Geometry: final body of the model. Coordinates: model frame, mm. A direction names the side the tool comes from. Coordinates: 2 decimals unless noted, no trailing zeros. Write each loop counter-clockwise with the first axis right and the second up, starting at its lowest first coordinate (ties: lowest second). Pieces come first, ordered by that corner, then holes. Notation, with made-up numbers: (70, 45) - (103, 45) arc R13 cw to (103, 60) - close; hole circle Ø4 at (-15, 44.25). An arc over 180 degrees is marked (long way). Put each result on its own line as item: value.
Autodesk Inventor part; units mm, degrees
ref_plane "YZ Plane" through (0, 0, 0) normal (1, 0, 0) x (0, 1, 0)
ref_plane "XZ Plane" through (0, 0, 0) normal (0, 1, 0) x (-1, 0, 0)
ref_plane "XY Plane" through (0, 0, 0) normal (0, 0, 1) x (1, 0, 0)
sketch "Sketch1" plane through (0, 0, 0) normal (0, 1, 0) x (-1, 0, 0)
  line L0 (-12.7612, -185.5673) -> (304.7388, -185.5673)
  line L1 (304.7388, -185.5673) -> (304.7388, 4.9327)
  line L2 (304.7388, 4.9327) -> (-12.7612, 4.9327)
  line L3 (-12.7612, 4.9327) -> (-12.7612, -185.5673)
  point P0 (0, 0)
  dimension "d0" = 317.5
  dimension "d1" = 190.5
extrude "Extrusion1" add sketch "Sketch1" along normal blind 1.5875
sketch "Sketch2" plane through (0, 1.5875, 0) normal (0, 1, 0) x (1, 0, 0)
  line L0 (12.7612, 185.5673) -> (-304.7388, 185.5673)
  line L1 (12.7612, -4.9327) -> (12.7612, 185.5673)
  line L2 (-341.3221, 147.4673) -> (43.4131, 147.4673)
  point P0 (0, 0)
  dimension "d4" = 38.1
bend part "Bend Part1" radius 2.54 angle 90 line through (-341.3221, 1.5875, -147.4673) along (1, 0, 0) centre toward (0, 1, 0) moving side (0, 0, -1) both sides no
properties part number "battery holder poly"
1. Section query A-A (x = -103.5). Return loops of the section in (y, z) (1 decimal).
Answer below:
outline: (0, -147.5) arc R4.1 ccw to (4.1, -151.6) - (38.2, -151.6) - (38.2, -150) - (4.1, -150) arc R2.5 cw to (1.6, -147.5) - (1.6, 4.9) - (0, 4.9) - close
2. Section query B-B (z = -97.5). Return loops of the section in (x, y), then the cut area to 3 significant figures.
Answer below:
outline: (-304.74, 0) - (12.76, 0) - (12.76, 1.59) - (-304.74, 1.59) - close
area: 504 mm²
3. Ray query, probe 1 along Z at (x, y) = (-164, 20); probe 2 along Y at (x, z) = (-277, -109.5); probe 3 along Z at (x, y) = (-288.5, 2). Return the intervals inside material, ascending. Write a range as from..to.
Answer below:
probe 1: z = -151.59..-150.01
probe 2: y = 0..1.59
probe 3: z = -151..-148.85
4. Set-up query: faces 1 (the flat face through (12.761, 1, -73)), 2 (the flat face through (-144, 21, -150.007)). Return all of +Z, -Z, +X, -X, +Y, -Y with unobstructed straight access to the full face (end or side cutting, diameter ignored); none if empty.
Answer below:
face 1: +Z, -Z, +X, +Y, -Y
face 2: +Z, +X, -X, +Y
5. Mould query, pull axis Y, two halves, no side actions, for faces 3 (the flat face through (-144, 0, -70)), 4 (the flat face through (-304.739, 1, -74)), 5 (the flat face through (-144, 1.588, -70)). Classes: +Y half, -Y half, draft (parallel to the pull), parting line (faces both ways), or undercut.
Answer below:
face 3: -Y half
face 4: draft
face 5: +Y half
6. Section query C-C (y = 21.5). Return loops of the section in (x, z).
Answer below:
outline: (-304.74, -151.59) - (12.76, -151.59) - (12.76, -150.01) - (-304.74, -150.01) - close
7. Pin query (flat end, axial travel): pin 1 Ø4 at (x, y) = (-215.5, 15) entering from +Z; pin 2 Ø12 at (x, z) = (-244.5, -78.5) entering from -Y; pin 3 Ø1.5 at (x, z) = (-202, -109.5) entering from +Y. Return the tip coordinate at first contact, or that it passes through.
Answer below:
pin 1: stops at z = -150.01
pin 2: stops at y = 0
pin 3: stops at y = 1.59
